For this review, use the dimensioned drawing (mm, ordinates from the lowest corner) and the shaded views. Coordinates: 2 decimals unless noted, no trailing zeros. Write each loop counter-clockwise with the first axis right and the second up, starting at its lowest first coordinate (ties: lowest second). Pieces come first, ordered by that corner, then holes.
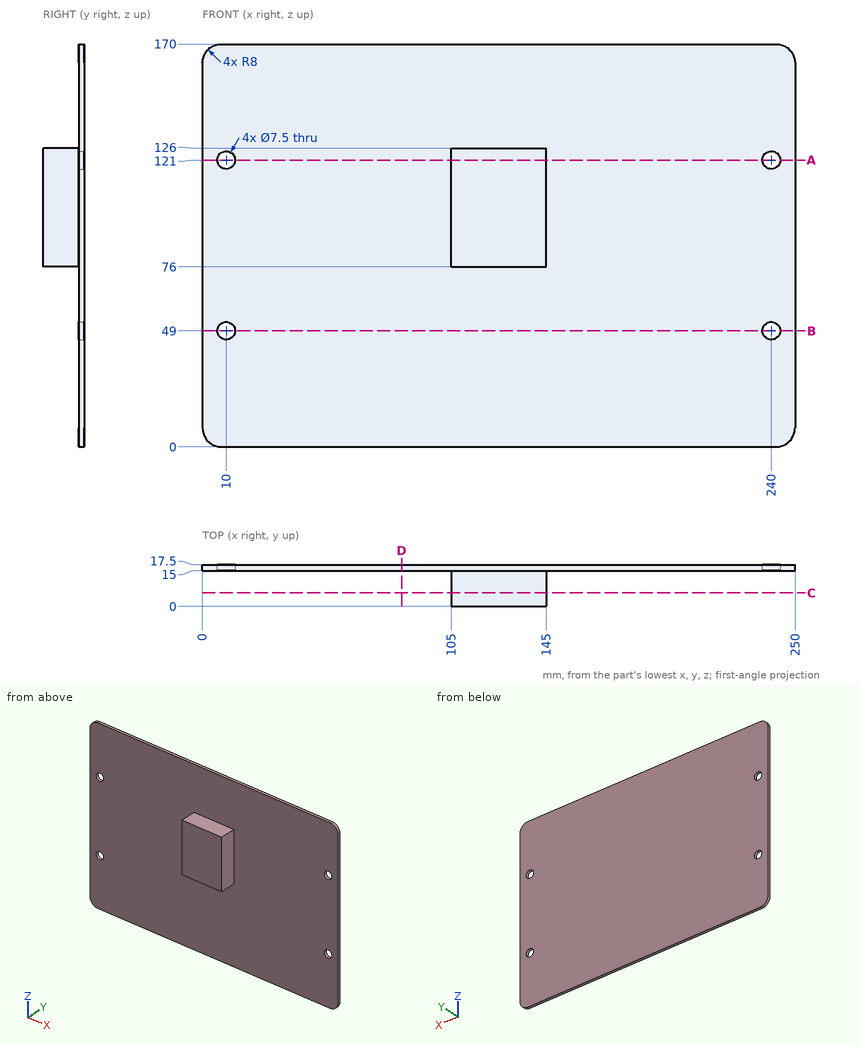
Item 1: Take a section at A-A, the plane z = 121. Write out the cut boundary in (x, y).
Solved:
outline: (0, 15) - (6.25, 15) - (6.25, 17.5) - (0, 17.5) - close; (13.75, 15) - (105, 15) - (105, 0) - (145, 0) - (145, 15) - (236.25, 15) - (236.25, 17.5) - (13.75, 17.5) - close; (243.75, 15) - (250, 15) - (250, 17.5) - (243.75, 17.5) - close
Item 2: Take a section at D-D, the plane x = 84. Write out the cut boundary in (y, z).
Solved:
outline: (15, 0) - (17.5, 0) - (17.5, 170) - (15, 170) - close
Item 3: Take a section at B-B, the plane z = 49. Write out the cut boundary in (x, y).
Solved:
outline: (0, 15) - (6.25, 15) - (6.25, 17.5) - (0, 17.5) - close; (13.75, 15) - (236.25, 15) - (236.25, 17.5) - (13.75, 17.5) - close; (243.75, 15) - (250, 15) - (250, 17.5) - (243.75, 17.5) - close
Item 4: To check wall thickness, follow line 1 along Z through (x, y) = (10, 15.7); line 2 along X through (y, z) = (16.15, 121); line 3 along X through (y, z) = (16, 47). State the ranges of each line that lie inside material, in increasing order.
Solved:
line 1: z = 0 to 45.25, 52.75 to 117.25, 124.75 to 170
line 2: x = 0 to 6.25, 13.75 to 236.25, 243.75 to 250
line 3: x = 0 to 6.83, 13.17 to 236.83, 243.17 to 250
Item 5: Take a section at C-C, the plane y = 5.75. Write out the cut boundary in (x, z).
Solved:
outline: (105, 76) - (145, 76) - (145, 126) - (105, 126) - close
Item 6: For pin 1 (4.5 mm diameter, centred on y = 5, z = 108, fed in from +X); pin 2 (4.5 mm diameter, centred on y = 4.5, z = 111.5, fed in from -X); pin 3 (5 mm diameter, centred on x = 61.5, z = 100.5, fed in from -Y); pin 4 (4.5 mm diameter, centred on x = 10, z = 49, fed in from +Y), all flat-tipped, find the tip position at first contact; note any pin that passes through.
Solved:
pin 1: stops at x = 145
pin 2: stops at x = 105
pin 3: stops at y = 15
pin 4: passes through
